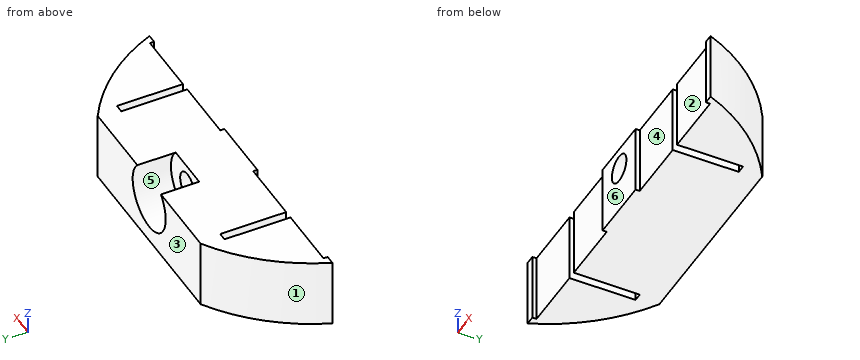
```python
from build123d import *

# Parameters (mm, degrees)
F1_DEPTH = 19.05
F3_R     = 2.794
F4_DEPTH = 18.258491
F5_R     = 6.35
F6_DEPTH = 7.62
F7_W     = 82.632937
F7_H     = 21.472244
F8_DEPTH = 5.08


with BuildPart() as f1:
    # F0 (on Top) → F1 (new body)
    with BuildSketch(Plane.XY):
        with BuildLine():
            Line((0, 32.303751), (-19.815022, 32.303751))
            ThreePointArc((-19.815022, 32.303751), (-28.981906, 24.417547), (-35.197985, 14.04526))
            Line((-35.197985, 14.04526), (-33.401, 14.04526))
            Line((-33.401, 14.04526), (-33.401, 14.87076))
            Line((-33.401, 14.87076), (-20.701, 14.87076))
            Line((-20.701, 14.87076), (-20.701, 28.01526))
            Line((-20.701, 28.01526), (-19.05, 28.01526))
            Line((-19.05, 28.01526), (-19.05, 14.87076))
            Line((-19.05, 14.87076), (-6.35, 14.87076))
            Line((-6.35, 14.87076), (-6.35, 14.04526))
            Line((-6.35, 14.04526), (0, 14.04526))
            Line((0, 14.04526), (0, 32.303751))
        make_face()
    extrude(amount=F1_DEPTH)

    # F2: F1 across plane


with BuildPart() as f1_1:
    add(f1.part)
    add(f1.part.mirror(Plane.YZ))

    # F3 (on face) → F4 (cut, through all)
    with BuildSketch(Plane(origin=(0, 32.303751, 0), x_dir=(-1, 0, 0), z_dir=(0, 1, 0))):
        with Locations((0, 9.525)):
            Circle(F3_R)
    extrude(amount=-F4_DEPTH, mode=Mode.SUBTRACT)

    # F5 (on face) → F6 (cut)
    with BuildSketch(Plane(origin=(0, 32.303751, 0), x_dir=(-1, 0, 0), z_dir=(0, 1, 0))):
        with Locations((0, 9.525)):
            Circle(F5_R)
    extrude(amount=-F6_DEPTH, mode=Mode.SUBTRACT)

    # F7 (on face) → F8 (cut)
    with BuildSketch(Plane.XY.offset(19.05)):
        with Locations((1.089636, 23.172186)):
            Rectangle(F7_W, F7_H)
    extrude(amount=-F8_DEPTH, mode=Mode.SUBTRACT)


solid = f1_1.part
```
Design review of the part built by this model. Coordinates are the model's own, in mm. Face numbers are marked on the shaded views. A direction names the side the tool comes from. Give positions to 0.01 mm unless a question says otherwise; leave off trailing zeros. Order: outer loops, then holes, each group sorted by start corner. A loop starts at its lowest first (then second) coordinate and runs counter-clockwise, first axis right, second up. Notation, with made-up numbers: (82.25, 88) - (119.25, 88) arc R24 cw to (119.25, 117) - close; hole circle Ø4 at (24.5, -16.5). An arc over 180 degrees is marked (long way). Use a Markdown table: item, result. Add a question column.
(1) Add section D-D on z = 11.25. Give the boundary of the cut face in (x, y).
(2) Add section B-B on y = 23.5. Give the boundary of the cut face in (x, z) (3 decimals), then the cut area to 3 significant figures.
(3) Mouldability with a two-part tool opening along X and no side actions: class the marked faces 1, 2 and 3 as +X half, -X half, draft (parallel to the pull), parting line (faces both ways), or undercut.
(4) Clearance check with flat-ended pins moving along their axes: P1, Ø1.3, axis at x = 20, z = 9, coming from the -Y side; P2, Ø6.5, axis at y = 19.5, z = 5, coming from the +X side; P3, Ø3, axis at x = -2, z = 7, coming from the +Y side. State where each tip first meets the part, or that it passes through.
(5) Wall thickness on probe 1 along X at (y, z) = (20.5, 2.75); probe 2 along X at (y, z) = (17.75, 8.5); probe 3 along X at (y, z) = (23.75, 8.25): over which ranges is each line inside the solid? List them lowest first. Write a range as [from, to].
(6) Add section A-A on x = 0. Give the boundary of the cut face in (y, z) (3 decimals).
(7) Add section C-C on z = 1.25. Give the boundary of the cut face in (x, y), then the cut area to 3 significant figures.
(8) Machinability: for the marked faces 4, 5 and 6, which of the approach directions +Z, -Z, +X, -X, +Y, -Y give a long, thin tool a straight path to every point of the face, cutting with its end or side? Answer none if there is none.
Report:
| question | item | result |
|---|---|---|
| 1 | outline | (-35.2, 14.05) - (-33.4, 14.05) - (-33.4, 14.87) - (-20.7, 14.87) - (-20.7, 28.02) - (-19.05, 28.02) - (-19.05, 14.87) - (-6.35, 14.87) - (-6.35, 14.05) - (-2.2, 14.05) - (-2.2, 24.68) - (-6.11, 24.68) - (-6.11, 32.3) - (-19.82, 32.3) arc R37.9 ccw to start; (2.2, 14.05) - (6.35, 14.05) - (6.35, 14.87) - (19.05, 14.87) - (19.05, 28.02) - (20.7, 28.02) - (20.7, 14.87) - (33.4, 14.87) - (33.4, 14.05) - (35.2, 14.05) arc R37.9 ccw to (19.82, 32.3) - (6.11, 32.3) - (6.11, 24.68) - (2.2, 24.68) - close |
| 2 | outline | (-29.731, 0) - (-20.701, 0) - (-20.701, 13.97) - (-29.731, 13.97) - close; (-19.05, 0) - (19.05, 0) - (19.05, 13.97) - (-19.05, 13.97) - close; (20.701, 0) - (29.731, 0) - (29.731, 13.97) - (20.701, 13.97) - close; hole circle Ø5.588 at (0, 9.525) |
| 2 | area | 760 mm² |
| 3 | face 1 | -X half |
| 3 | face 2 | undercut |
| 3 | face 3 | draft |
| 4 | P1 | stops at y = 28.02 |
| 4 | P2 | stops at x = 34.24 |
| 4 | P3 | stops at y = 24.68 |
| 5 | probe 1 | x = [-31.87, -20.7], [-19.05, 19.05], [20.7, 31.87] |
| 5 | probe 2 | x = [-33.48, -20.7], [-19.05, -2.6], [2.6, 19.05], [20.7, 33.48] |
| 5 | probe 3 | x = [-29.53, -20.7], [-19.05, -2.49], [2.49, 19.05], [20.7, 29.53] |
| 6 | outline | (14.045, 0) - (32.304, 0) - (32.304, 3.175) - (24.684, 3.175) - (24.684, 6.731) - (14.045, 6.731) - close; (14.045, 12.319) - (24.684, 12.319) - (24.684, 13.97) - (14.045, 13.97) - close |
| 7 | outline | (-35.2, 14.05) - (-33.4, 14.05) - (-33.4, 14.87) - (-20.7, 14.87) - (-20.7, 28.02) - (-19.05, 28.02) - (-19.05, 14.87) - (-6.35, 14.87) - (-6.35, 14.05) - (6.35, 14.05) - (6.35, 14.87) - (19.05, 14.87) - (19.05, 28.02) - (20.7, 28.02) - (20.7, 14.87) - (33.4, 14.87) - (33.4, 14.05) - (35.2, 14.05) arc R37.9 ccw to (19.82, 32.3) - (-19.82, 32.3) arc R37.9 ccw to start |
| 7 | area | 978 mm² |
| 8 | face 4 | +Z, -Z, -Y |
| 8 | face 5 | +Y |
| 8 | face 6 | +Z, -Z, +X, -X, -Y |
